Geometry: see drawing. Coordinates: mm, zero at the bounding-box minimum. Give positions to 0.01 mm unless a question says otherwise; leave off trailing zeros. Write each loop counter-clockwise with the first axis right and the second up, starting at its lowest first coordinate (ties: lowest second). Pieces come first, ordered by that corner, then holes. Notation, with made-up numbers: (57.5, 6) - (109.5, 6) arc R22 ccw to (109.5, 20) - close; hole circle Ø11 at (40, 56.5). An arc over 180 degrees is marked (long way). Use CSV: the item, a comma, the result in double quotes. Start each with the question number.
(1) Section C-C on y = 3.9. Output: boundary loops of the cut face in (x, z), and give its area (3 significant figures).
(2) Draft query along Z for the marked faces 1, 2 and 3. Return one class per face: released by +Z, released by -Z, zero draft, split by the parting line, or undercut.
(3) First-contact query: pin 1 Ø2 at (y, z) = (1.5, 20.5) entering from +X; pin 2 Ø1 at (x, y) = (9, 1) entering from +Z (1 decimal); pin 3 Ø5 at (x, z) = (24, 35) entering from +Y. Flat tips, straight axial feed; report the tip coordinate or a pass-through.
(4) Line query: probe 1 along Z at (x, y) = (25, 4); probe 2 along X at (y, z) = (0.75, 35); probe 3 along Z at (x, y) = (15.5, 0.4) (1 decimal). Output: solid intervals per line, ascending. Write a range as [from, to].
(5) Section A-A on x = 35. Output: boundary loops of the cut face in (y, z), and give its area (3 significant figures).
(6) Section D-D on x = 25. Output: boundary loops of the cut face in (y, z).
(7) Section B-B on z = 25. Output: boundary loops of the cut face in (x, y), and give its area (3 significant figures).
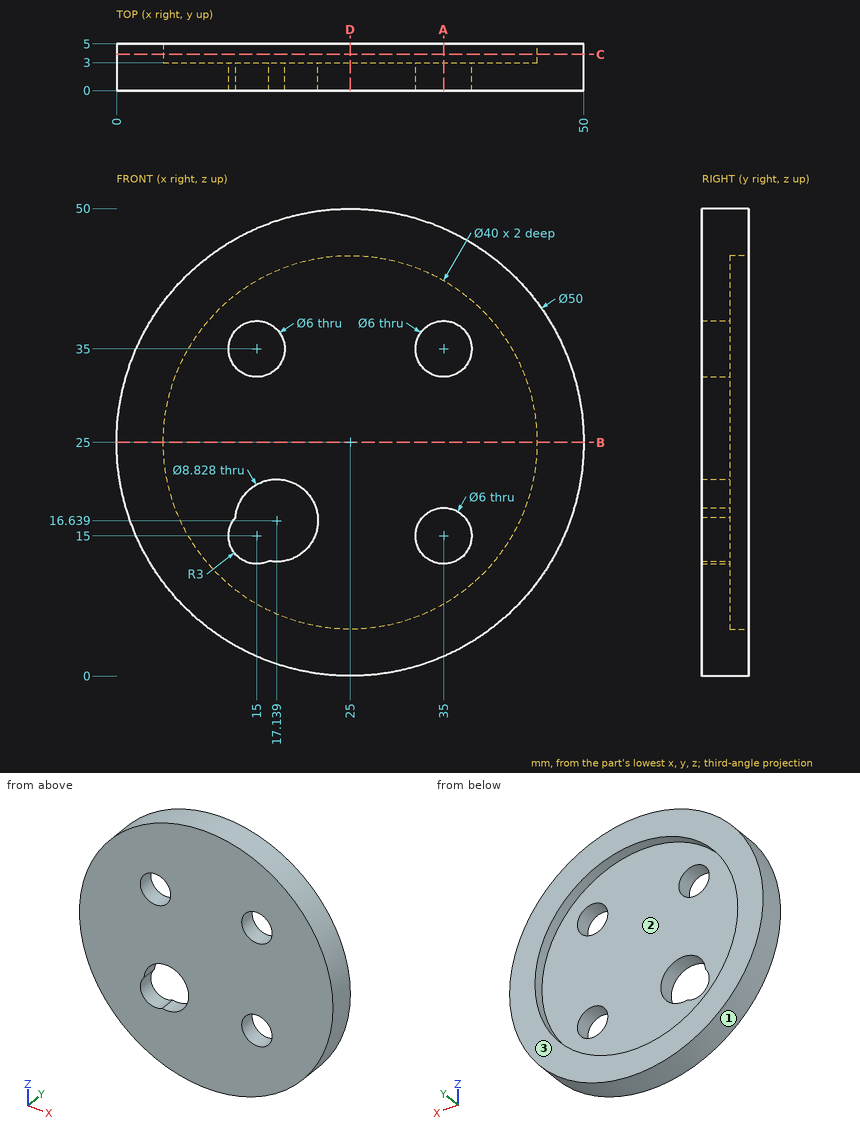
Check values:
1,outline,"circle Ø50 at (25, 25); hole circle Ø40 at (25, 25)"
1,area,"707 mm²"
2,face 1,"split by the parting line"
2,face 2,"undercut"
2,face 3,"zero draft"
3,pin 1,"stops at x = 49.75"
3,pin 2,"stops at z = 44.6"
3,pin 3,"stops at y = 3"
4,probe 1,"z = [0, 5], [45, 50]"
4,probe 2,"x = [2.09, 12], [18, 32], [38, 47.91]"
4,probe 3,"z = [1.9, 12], [20.7, 32], [38, 48.1]"
5,outline,"(0, 2.09) - (5, 2.09) - (5, 7.68) - (3, 7.68) - (3, 12) - (0, 12) - close; (0, 18) - (3, 18) - (3, 32) - (0, 32) - close; (0, 38) - (3, 38) - (3, 42.32) - (5, 42.32) - (5, 47.91) - (0, 47.91) - close"
5,area,"124 mm²"
6,outline,"(0, 0) - (5, 0) - (5, 5) - (3, 5) - (3, 45) - (5, 45) - (5, 50) - (0, 50) - close"
7,outline,"(0, 0) - (50, 0) - (50, 5) - (45, 5) - (45, 3) - (5, 3) - (5, 5) - (0, 5) - close"
7,area,"170 mm²"
